Read the model definition and answer for the solid it produces. Units are mm, in the model's axes. Face numbers are marked on the shaded views. A direction names the side the tool comes from. Coordinates: 2 decimals unless noted, no trailing zeros. Write each loop counter-clockwise with the first axis right and the second up, starting at its lowest first coordinate (ties: lowest second). Pieces come first, ordered by that corner, then holes.
(1) The mould has two halves that part along X. Classify the marked faces 4, 5 and 6: +X half, -X half, draft (parallel to the pull), parting line (faces both ways), or undercut.
(2) Section D-D on y = 2.5 is taken. Write down the section's boundary in (x, z), then the cut area to 3 significant figures.
(3) Section A-A on x = 0 is taken. Write down the section's boundary in (y, z).
(4) Section B-B on z = 0 is taken. Write down the section's boundary in (x, y), then the cut area to 3 significant figures.
(5) Section C-C on y = 3.95 is taken. Write down the section's boundary in (x, z), then the cut area to 3 significant figures.
(6) Find the intervals of material crossed by probe 1 along X at (y, z) = (4.05, 0); probe 2 along X at (y, z) = (1.45, -0.05); probe 3 along Y at (x, z) = (-1.85, 0.55), in increasing order.
(7) Which of the six approach directions +Z, -Z, +X, -X, +Y, -Y give full straight-line access (tool end or side, diameter ignored) to the marked faces 1, 2 and 3?
(8) Given pin 1 (1.9 mm diameter, centred on x = -0.5, z = 0.5, fed in from -Y); pin 2 (2 mm diameter, centred on x = 0, y = 0.5, fed in from +Z); pin 3 (2 mm diameter, centred on x = -0.5, z = 0.5, fed in from +Y), each flat-ended and moving along its own axis, determine where each tip first touches the part or whether it passes through.
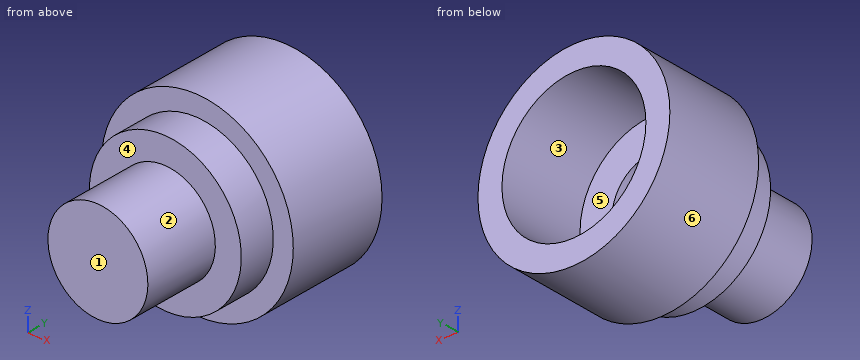
from build123d import *

# Parameters (mm, degrees)
SKETCH1_R           = 1.25
BOSS_EXTRUDE1_DEPTH = 1.9
SKETCH2_R           = 1.9
BOSS_EXTRUDE2_DEPTH = 0.9
SKETCH4_R           = 2.4
BOSS_EXTRUDE4_DEPTH = 2.5
SKETCH6_R           = 1.8
CUT_EXTRUDE2_DEPTH  = 2.2
SKETCH5_R           = 1
CUT_EXTRUDE1_DEPTH  = 2.9


with BuildPart() as part:
    # Sketch1 → Boss-Extrude1 (new body)
    with BuildSketch(Plane(origin=(0, 0, 0), x_dir=(1, 0, 0), z_dir=(0, 1, 0))):
        with Locations(Location((0, 0, 0), (0, 0, 90))):
            Circle(SKETCH1_R)
    extrude(amount=BOSS_EXTRUDE1_DEPTH)

    # Sketch2 → Boss-Extrude2 (add)
    with BuildSketch(Plane(origin=(0, 1.9, 0), x_dir=(1, 0, 0), z_dir=(0, 1, 0))):
        with Locations(Location((0, 0, 0), (0, 0, 270))):
            Circle(SKETCH2_R)
    extrude(amount=BOSS_EXTRUDE2_DEPTH)

    # Sketch4 → Boss-Extrude4 (add)
    with BuildSketch(Plane(origin=(0, 5.3, 0), x_dir=(1, 0, 0), z_dir=(0, 1, 0))):
        with Locations(Location((0, 0, 0), (0, 0, 270))):
            Circle(SKETCH4_R)
    extrude(amount=-BOSS_EXTRUDE4_DEPTH)

    # Sketch6 → Cut-Extrude2 (cut)
    with BuildSketch(Plane(origin=(0, 5.3, 0), x_dir=(1, 0, 0), z_dir=(0, 1, 0))):
        with Locations(Location((0, 0, 0), (0, 0, 270))):
            Circle(SKETCH6_R)
    extrude(amount=-CUT_EXTRUDE2_DEPTH, mode=Mode.SUBTRACT)

    # Sketch5 → Cut-Extrude1 (cut)
    with BuildSketch(Plane(origin=(0, 3.1, 0), x_dir=(1, 0, 0), z_dir=(0, 1, 0))):
        with Locations(Location((0, 0, 0), (0, 0, 270))):
            Circle(SKETCH5_R)
    extrude(amount=-CUT_EXTRUDE1_DEPTH, mode=Mode.SUBTRACT)


solid = part.part
Response:
1. face 4: draft
1. face 5: undercut
1. face 6: parting line
2. outline: circle Ø3.8 at (0, 0); hole circle Ø2 at (0, 0)
2. area: 8.20 mm2
3. outline: (0, -1.25) - (1.9, -1.25) - (1.9, -1.9) - (2.8, -1.9) - (2.8, -2.4) - (5.3, -2.4) - (5.3, -1.8) - (3.1, -1.8) - (3.1, -1) - (0.2, -1) - (0.2, 1) - (3.1, 1) - (3.1, 1.8) - (5.3, 1.8) - (5.3, 2.4) - (2.8, 2.4) - (2.8, 1.9) - (1.9, 1.9) - (1.9, 1.25) - (0, 1.25) - close
4. outline: (-2.4, 2.8) - (-1.9, 2.8) - (-1.9, 1.9) - (-1.25, 1.9) - (-1.25, 0) - (1.25, 0) - (1.25, 1.9) - (1.9, 1.9) - (1.9, 2.8) - (2.4, 2.8) - (2.4, 5.3) - (1.8, 5.3) - (1.8, 3.1) - (1, 3.1) - (1, 0.2) - (-1, 0.2) - (-1, 3.1) - (-1.8, 3.1) - (-1.8, 5.3) - (-2.4, 5.3) - close
4. area: 6.45 mm2
5. outline: circle Ø4.8 at (0, 0); hole circle Ø3.6 at (0, 0)
5. area: 7.92 mm2
6. probe 1: x = -2.4 to -1.8, 1.8 to 2.4
6. probe 2: x = -1.25 to -1, 1 to 1.25
6. probe 3: y = 2.8 to 5.3
7. face 1: +Z, -Z, +X, -X, -Y
7. face 2: -Y
7. face 3: +Y
8. pin 1: stops at y = 0
8. pin 2: stops at z = 1.25
8. pin 3: stops at y = 3.1
